from build123d import *

# Parameters (mm, degrees)
F0_W     = 30
F0_H     = 30
F0_R     = 3
F1_DEPTH = 5
F2_W     = 30
F2_H     = 35
F3_DEPTH = 5
F6_DEPTH = 2.5
F7_SIZE  = 5
F8_SIZE  = 2


with BuildPart() as f1:
    # F0 (on Top) → F1 (new body)
    with BuildSketch(Plane.XY):
        with Locations((-89.0373364091, 8)):
            Rectangle(F0_W, F0_H)
        with Locations((-89.0373364091, 0)):
            Circle(F0_R, mode=Mode.SUBTRACT)
        with Locations((-89.0373364091, 16)):
            Circle(F0_R, mode=Mode.SUBTRACT)
    extrude(amount=F1_DEPTH)

    # F2 (on face) → F3 (join)
    with BuildSketch(Plane(origin=(-104.0373364091, 0, 0), x_dir=(0, -1, 0), z_dir=(-1, 0, 0))):
        with Locations((-8, 22.5)):
            Rectangle(F2_W, F2_H)
    extrude(amount=-F3_DEPTH)

    # F5 (on line) → F6 (join, symmetric)
    with BuildSketch(Plane(origin=(0, 8, 0), x_dir=(-1, 0, 0), z_dir=(0, 1, 0))):
        Polygon((99.0373364091, 5), (99.0373364091, 40), (74.0373364091, 5), align=None)
    extrude(amount=F6_DEPTH, both=True)

    # F7
    f7_edges = [f1.edges().sort_by_distance(p)[0] for p in [
        (-101.537336, -7, 40),
        (-101.537336, 23, 40),
        (-74.037336, -7, 2.5),
        (-74.037336, 23, 2.5),
    ]]
    chamfer(f7_edges, length=F7_SIZE)

    # F8
    f8_edges = [f1.edges().sort_by_distance(p)[0] for p in [
        (-92.037336, 0, 5),
        (-92.037336, 16, 5),
    ]]
    chamfer(f8_edges, length=F8_SIZE)


solid = f1.part
Read the model definition and answer for the solid it produces. Units are mm, in the model's axes. A direction names the side the tool comes from. Coordinates: 2 decimals unless noted, no trailing zeros. Loops run counter-clockwise (first coordinate to the right, second up) from the corner with the lowest first, then second, coordinate; pieces in that order, holes last.
Q1. Each of these flat-tipped pins is pushed along its axis until it touches: pin 1 Ø1.5 at (x, y) = (-79, 1) entering from +Z; pin 2 Ø7.5 at (x, z) = (-85.5, 21) entering from +Y; pin 3 Ø10 at (x, z) = (-78.5, 16) entering from -Y; pin 4 Ø1 at (x, y) = (-97, -0.5) entering from -Z. Where does it stop, or does it pass through?
Q2. Which of the six approach directions +Z, -Z, +X, -X, +Y, -Y give full straight-line access (tool end or side, diameter ignored) to faces 4 (the face through (-92, 5.5, 15)), 5 (the face through (-83.9, 16.8, 5)), 6 (the face through (-102, -5, 37))?
Q3. The part is cut by section B-B on z = 19.5. Write down the section's boundary in (x, y).
Q4. The part is cut by section A-A on y = 16. Write down the section's boundary in (x, z).
Q5. The part is cut by section C-C on x = -88.5. Give the number of separate pieces and of enclosed holes in the cut face, and give its area (3 significant figures).
Q6. The mould has two halves that part along X. Classify faces 1 (the face through (-74.037, 8, 2)), 2 (the face through (-92, 10.5, 15)), 3 (the face through (-86.057, 0.939, 3.125)): +X half, -X half, draft (parallel to the pull), parting line (faces both ways), or undercut.
Q7. The part is cut by section D-D on x = -78.5. Write down the section's boundary in (y, z).
Q8. Consider probe 1 along Z at (x, y) = (-83.25, 1.25); probe 2 along X at (y, z) = (11, 26); probe 3 along X at (y, z) = (19.5, 4.5). Determine where each line is inside the solid, lowest interval first.
Results below:
1. pin 1: stops at z = 5
1. pin 2: stops at y = 10.5
1. pin 3: stops at y = 5.5
1. pin 4: stops at z = 0
2. face 4: +Z, +X, -Y
2. face 5: +Z, +X, +Y
2. face 6: +Z, +X, -X, -Y
3. outline: (-104.04, -7) - (-99.04, -7) - (-99.04, 5.5) - (-84.39, 5.5) - (-84.39, 10.5) - (-99.04, 10.5) - (-99.04, 23) - (-104.04, 23) - close
4. outline: (-104.04, 0) - (-92.04, 0) - (-92.04, 3) - (-94.04, 5) - (-99.04, 5) - (-99.04, 40) - (-104.04, 40) - close; (-86.04, 0) - (-74.04, 0) - (-74.04, 5) - (-84.04, 5) - (-86.04, 3) - close
5. separate pieces: 3
5. enclosed holes: 0
5. area: 184 mm2
6. face 1: +X half
6. face 2: draft
6. face 3: undercut
7. outline: (-6.46, 0) - (22.46, 0) - (22.46, 5) - (10.5, 5) - (10.5, 11.25) - (5.5, 11.25) - (5.5, 5) - (-6.46, 5) - close
8. probe 1: z = 0 to 5
8. probe 2: x = -104.04 to -99.04
8. probe 3: x = -104.04 to -91.87, -86.21 to -75.54
